The model under review builds one solid part; all positions refer to its coordinate system, in mm. A direction names the side the tool comes from. Coordinates: 2 decimals unless noted, no trailing zeros. Loops run counter-clockwise (first coordinate to the right, second up) from the corner with the lowest first, then second, coordinate; pieces in that order, holes last. Notation, with made-up numbers: M -21,-25 L 16,-25 A12 cw 16,-16 Z; hole C 35.25,49.5 d3. An arc over 180 degrees is marked long. Return JSON: item names as keys, results as strings.
```python
from build123d import *

# Parameters (mm, degrees)
F0_W        = 150
F0_H        = 25
F1_DEPTH    = 3
F2_W        = 100
F2_H        = 2
F3_DEPTH    = 7
F4_W        = 42
F4_H        = 5.5
F4_H_2      = 29.5
F5_DEPTH    = 11
F5_TAPER    = -30
F6_W        = 75
F6_H        = 3
F7_DEPTH    = 7.001
F8_T1_DEPTH = 47.9128784748


# Not quite as in the source:
# - a fillet or chamfer that OpenCascade refuses, or shapes differently, is made with other operations: its cross-section is extruded or revolved along the edge and cut away or added


with BuildPart() as f1:
    # F0 (on Top) → F1 (new body)
    with BuildSketch(Plane.XY):
        with Locations((75, 12.5)):
            Rectangle(F0_W, F0_H)
    extrude(amount=F1_DEPTH)

    # F2 (on Top) → F3 (join)
    with BuildSketch(Plane.XY):
        with Locations((50, 24)):
            Rectangle(F2_W, F2_H)
        with Locations((50, 1)):
            Rectangle(F2_W, F2_H)
    extrude(amount=F3_DEPTH)

    # F4 (on Top) → F5 (join)
    with BuildSketch(Plane.XY):
        with Locations((129, -2.75)):
            Rectangle(F4_W, F4_H)
        with Locations((129, 14.75)):
            Rectangle(F4_W, F4_H_2)
    extrude(amount=-F5_DEPTH, taper=F5_TAPER)

    # F6 (on Top) → F7 (cut, through all)
    with BuildSketch(Plane.XY):
        with Locations((52.5, 12.5)):
            Rectangle(F6_W, F6_H)
    extrude(amount=F7_DEPTH, mode=Mode.SUBTRACT)

    # F8: fillet of radius 5 on 1 edges, made by hand

    # F8_s2 → F8_t1 (cut)
    with BuildSketch(Plane.XZ.offset(-36.4564392374)):
        with BuildLine():
            ThreePointArc((145.417424305, 3), (148.1560370926, 2.1833001327), (150, 0))
            Line((150, 0), (150.0916515139, 0.04))
            ThreePointArc((150.0916515139, 0.04), (150.1, 1.5), (150.1, 3))
            Line((150.1, 3), (150, 3.1))
            Line((150, 3.1), (145.417424305, 3.1))
            Line((145.417424305, 3.1), (145.417424305, 3))
        make_face()
    extrude(amount=F8_T1_DEPTH, mode=Mode.SUBTRACT)


solid = f1.part
```
1. Add section A-A on x = 40.5. Give the boundary of the cut face in (y, z).
Check values:
{"outline": "M 0,0 L 11,0 L 11,3 L 2,3 L 2,7 L 0,7 Z; M 14,0 L 25,0 L 25,7 L 23,7 L 23,3 L 14,3 Z"}
2. To check wall thickness, follow line 1 (Y direction, x = 85.5, z = 2.75); line 2 (Y direction, x = 94, z = 6.25); line 3 (Z direction, x = 137.5, y = -1.5). State the ranges of each line that lie inside material, in increasing order.
Check values:
{"line 1": "0 to 11, 14 to 25", "line 2": "0 to 2, 23 to 25", "line 3": "-11 to 0"}
3. Insertion check: pin 1 Ø4 at (x, z) = (35.5, 1) entering from -Y; pin 2 Ø2.5 at (x, z) = (42.5, 1) entering from +Y; pin 3 Ø6 at (x, y) = (110, 15.5) entering from +Z. Each pin has a flat end and moves straight along its axis. Give the tip position at first contact, or say it passes through.
Check values:
{"pin 1": "y = 0", "pin 2": "y = 25", "pin 3": "z = 3"}
4. The part is to be moulded in two halves that separate along X. For faces 5 (the face through (57, 0, 3)), 6 (the face through (0, 12, 2)), 7 (the face through (148.122, 12.675, 2.205)), 8 (the face through (52, 14, 1)), say which applies: released by +X, released by -X, zero draft, split by the parting line, or undercut.
Check values:
{"face 5": "zero draft", "face 6": "released by -X", "face 7": "released by +X", "face 8": "undercut"}
5. Add section B-B on x = 11.5. Give the boundary of the cut face in (y, z), plus the area to 3 significant figures.
Check values:
{"outline": "M 0,0 L 25,0 L 25,7 L 23,7 L 23,3 L 2,3 L 2,7 L 0,7 Z", "area": "91.0 mm²"}
6. Machinability: for faces 1 (the face through (129, 27, 0)), 2 (the face through (90, 12, 1)), 3 (the face through (49, 23, 5)), 4 (the face through (128, -2, 0)), which of the approach directions +Z, -Z, +X, -X, +Y, -Y give a long, thin tool a straight path to every point of the face, cutting with its end or side? Answer none if there is none.
Check values:
{"face 1": "+Z, +X, -X, +Y", "face 2": "+Z, -Z", "face 3": "+Z, +X, -X", "face 4": "+Z, +X, -X, -Y"}
